Check sheet for the modelled part. Datum: model origin and axes. Units: mm. Face numbers are marked on the shaded views. Round coordinates to 2 decimals unless told otherwise and drop trailing zeros. Loops run counter-clockwise (first coordinate to the right, second up) from the corner with the lowest first, then second, coordinate; pieces in that order, holes last. Notation, with made-up numbers: M 55.5,63 L 80.5,63 A30 ccw 80.5,98 Z; hole C -29.75,58 d4. An arc over 180 degrees is marked long. One line per question, with ' | ' between items. Start each with the question number.
(1) Section check C-C (y = -41.5). Record the boundary of the cut face in (x, z), and give its area (3 significant figures).
(2) Go/stop test with flat-tipped pins: P1, Ø3, axis at x = 6.5, z = 35, coming from the +Y side; P2, Ø6.5, axis at x = 1.5, z = -1, coming from the -Y side; P3, Ø4, axis at x = 39, y = -3, coming from the +Z side; P4, Ø20.5, axis at x = 38.1, y = 0, coming from the +Z side. Record where each tip stops, or that it passes through.
(3) Draft check along X on the marked faces 1, 2 and 3. Enter one of: +X half, -X half, draft (parallel to the pull), parting line (faces both ways), or undercut.
(4) Thickness scan on probe 1 along Y at (x, z) = (0, 69); probe 2 along Y at (x, z) = (0, 0); probe 3 along Z at (x, y) = (0, -44). Record the ranges inside material, lowest first. Write a range as [from, to].
(5) Section check B-B (y = 0). Record the boundary of the cut face in (x, z).
(6) Section check D-D (z = 0). Record the boundary of the cut face in (x, y).
(7) Section check A-A (x = 0). Record the boundary of the cut face in (y, z), and give its area (3 significant figures).
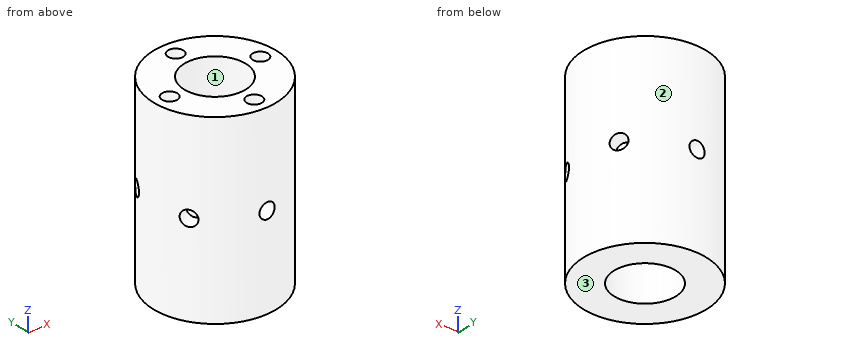
```python
from build123d import *

# Parameters (mm, degrees)
F0_W      = 50.8
F0_H      = 152.4
F3_R      = 6.35
F4_DEPTH  = 12.7
F5_COUNT  = 6
F8_R      = 25.4
F9_DEPTH  = 152.4
F12_R     = 6.35
F13_DEPTH = 25.4
F14_COUNT = 4


with BuildPart() as f1:
    # F0 (on Front) → F1 (revolve)
    with BuildSketch(Plane.XZ):
        with Locations((-25.4, 0)):
            Rectangle(F0_W, F0_H)
    revolve(axis=Axis((0, 0, 0), (0, 0, -1)))


with BuildPart() as f4:
    # F3 (on offset) → F4 (new body)
    with BuildSketch(Plane.XZ.offset(50.8)):
        Circle(F3_R)
    extrude(amount=-F4_DEPTH)


with BuildPart() as f5_1:
    # F5: instance of F4
    add(f4.part.rotate(Axis((0, 0, -76.2), (0, 0, -1)), 1 * 360 / F5_COUNT))


with BuildPart() as f5_2:
    # F5: instance of F4
    add(f4.part.rotate(Axis((0, 0, -76.2), (0, 0, -1)), 2 * 360 / F5_COUNT))


with BuildPart() as f5_3:
    # F5: instance of F4
    add(f4.part.rotate(Axis((0, 0, -76.2), (0, 0, -1)), 3 * 360 / F5_COUNT))


with BuildPart() as f5_4:
    # F5: instance of F4
    add(f4.part.rotate(Axis((0, 0, -76.2), (0, 0, -1)), 4 * 360 / F5_COUNT))


with BuildPart() as f5_5:
    # F5: instance of F4
    add(f4.part.rotate(Axis((0, 0, -76.2), (0, 0, -1)), 5 * 360 / F5_COUNT))


with BuildPart() as f1_1:
    add(f1.part)

    # F6: cut F4, F5_1, F5_2, F5_3, F5_4, F5_5
    add(f4.part, mode=Mode.SUBTRACT)
    add(f5_1.part, mode=Mode.SUBTRACT)
    add(f5_2.part, mode=Mode.SUBTRACT)
    add(f5_3.part, mode=Mode.SUBTRACT)
    add(f5_4.part, mode=Mode.SUBTRACT)
    add(f5_5.part, mode=Mode.SUBTRACT)


with BuildPart() as f9:
    # F8 (on offset) → F9 (new body)
    with BuildSketch(Plane.XY.offset(76.2)):
        Circle(F8_R)
    extrude(amount=-F9_DEPTH)


with BuildPart() as f1_2:
    add(f1_1.part)

    # F10: cut F9
    add(f9.part, mode=Mode.SUBTRACT)


with BuildPart() as f13:
    # F12 (on offset) → F13 (new body)
    with BuildSketch(Plane.XY.offset(76.2)):
        with Locations((0, 38.1)):
            Circle(F12_R)
    extrude(amount=-F13_DEPTH)


with BuildPart() as f14_1:
    # F14: instance of F13
    add(f13.part.rotate(Axis((0, 0, 0), (0, 0, -1)), 1 * 360 / F14_COUNT))


with BuildPart() as f14_2:
    # F14: instance of F13
    add(f13.part.rotate(Axis((0, 0, 0), (0, 0, -1)), 2 * 360 / F14_COUNT))


with BuildPart() as f14_3:
    # F14: instance of F13
    add(f13.part.rotate(Axis((0, 0, 0), (0, 0, -1)), 3 * 360 / F14_COUNT))


with BuildPart() as f1_3:
    add(f1_2.part)

    # F15: cut F13, F14_1, F14_2, F14_3
    add(f13.part, mode=Mode.SUBTRACT)
    add(f14_1.part, mode=Mode.SUBTRACT)
    add(f14_2.part, mode=Mode.SUBTRACT)
    add(f14_3.part, mode=Mode.SUBTRACT)


solid = f1_3.part
```
The answers:
1) outline: M -29.3,-76.2 L 29.3,-76.2 L 29.3,76.2 L 5.36,76.2 L 5.36,50.8 L -5.36,50.8 L -5.36,76.2 L -29.3,76.2 Z; hole C 0,0 d12.7 | area: 8,530 mm²
2) P1: y = 50.55 | P2: y = -38.1 | P3: z = 50.8 | P4: z = 76.2
3) face 1: undercut | face 2: parting line | face 3: draft
4) probe 1: [-50.8, -44.45], [-31.75, -25.4], [25.4, 31.75], [44.45, 50.8] | probe 2: [-38.1, -25.4], [25.4, 38.1] | probe 3: [-76.2, -6.35], [6.35, 50.8]
5) outline: M -50.8,-76.2 L -25.4,-76.2 L -25.4,76.2 L -31.75,76.2 L -31.75,50.8 L -44.45,50.8 L -44.45,76.2 L -50.8,76.2 Z; M 25.4,-76.2 L 50.8,-76.2 L 50.8,76.2 L 44.45,76.2 L 44.45,50.8 L 31.75,50.8 L 31.75,76.2 L 25.4,76.2 Z
6) outline: M -46.82,-19.7 L -36.17,-13.55 L -29.82,-24.55 L -40.47,-30.7 A50.8 ccw -6.35,-50.4 L -6.35,-38.1 L 6.35,-38.1 L 6.35,-50.4 A50.8 ccw 40.47,-30.7 L 29.82,-24.55 L 36.17,-13.55 L 46.82,-19.7 A50.8 ccw 46.82,19.7 L 36.17,13.55 L 29.82,24.55 L 40.47,30.7 A50.8 ccw 6.35,50.4 L 6.35,38.1 L -6.35,38.1 L -6.35,50.4 A50.8 ccw -40.47,30.7 L -29.82,24.55 L -36.17,13.55 L -46.82,19.7 A50.8 ccw Z; hole C 0,0 d50.8
7) outline: M -50.8,-76.2 L -25.4,-76.2 L -25.4,76.2 L -31.75,76.2 L -31.75,50.8 L -44.45,50.8 L -44.45,76.2 L -50.8,76.2 L -50.8,6.35 L -38.1,6.35 L -38.1,-6.35 L -50.8,-6.35 Z; M 25.4,-76.2 L 50.8,-76.2 L 50.8,-6.35 L 38.1,-6.35 L 38.1,6.35 L 50.8,6.35 L 50.8,76.2 L 44.45,76.2 L 44.45,50.8 L 31.75,50.8 L 31.75,76.2 L 25.4,76.2 Z | area: 6,770 mm²
